```python
from build123d import *

# Parameters (mm, degrees)
BOSS_EXTRUDE1_DEPTH                = 25.4
FILLET1_R                          = 25.4
F_1_4_0_25_DIAMETER_SLOT1_DEPTH    = 25.4
F_1_16_0_0625_DIAMETER_HOLE1_D     = 1.5875
F_1_16_0_0625_DIAMETER_HOLE1_DEPTH = 12.7
F_1_16_0_0625_DIAMETER_HOLE1_TIP   = 0.476933116


# Read off the part's stored shape, not the designer's step: 1/4 (0.25) Diameter Slot1
with BuildPart() as part:
    # Sketch1 → Boss-Extrude1 (new body)
    with BuildSketch(Plane.XY):
        Polygon((-203.2, 0), (203.2, 0), (173.589463707, -63.5), (-173.589463707, -63.5), align=None)
    extrude(amount=BOSS_EXTRUDE1_DEPTH)

    # Fillet1
    fillet1_edges = [part.edges().sort_by_distance(p)[0] for p in [
        (173.589463707, -63.5, 12.7),
        (-173.589463707, -63.5, 12.7),
    ]]
    fillet(fillet1_edges, radius=FILLET1_R)

    # 1/4 (0.25) Diameter Slot1 outline → 1/4 (0.25) Diameter Slot1 (cut)
    with BuildSketch(Plane.XY):
        with BuildLine():
            Line((-149.225, -41.275), (149.225, -41.275))
            ThreePointArc((149.225, -41.275), (152.4, -38.1), (149.225, -34.925))
            Line((149.225, -34.925), (-149.225, -34.925))
            ThreePointArc((-149.225, -34.925), (-152.4, -38.1), (-149.225, -41.275))
        make_face()
    extrude(amount=F_1_4_0_25_DIAMETER_SLOT1_DEPTH, mode=Mode.SUBTRACT)

    # 1/16 (0.0625) Diameter Hole1
    with Locations(Plane(origin=(0, 0, 0), x_dir=(1, 0, 0), z_dir=(0, 1, 0))):
        with Locations((-152.4, -12.7), (-101.6, -12.7), (-50.8, -12.7), (0, -12.7), (50.8, -12.7), (101.6, -12.7), (152.4, -12.7)):
            Hole(F_1_16_0_0625_DIAMETER_HOLE1_D / 2, depth=F_1_16_0_0625_DIAMETER_HOLE1_DEPTH)
            with Locations((0, 0, -(F_1_16_0_0625_DIAMETER_HOLE1_DEPTH + F_1_16_0_0625_DIAMETER_HOLE1_TIP / 2))):  # 118° drill point
                Cone(0, F_1_16_0_0625_DIAMETER_HOLE1_D / 2, F_1_16_0_0625_DIAMETER_HOLE1_TIP, mode=Mode.SUBTRACT)


solid = part.part
```
Input: part model. Units: mm. Frame: model coordinates. A direction names the side the tool comes from. Give positions to 0.01 mm unless a question says otherwise; leave off trailing zeros. Order: outer loops, then holes, each group sorted by start corner. A loop starts at its lowest first (then second) coordinate and runs counter-clockwise, first axis right, second up. Notation, with made-up numbers: M 1.5,-17.75 L 60.5,-17.75 A12 cw 60.5,-1.75 Z; hole C 87.5,14 d2. An arc over 180 degrees is marked long. One line per question, with ' | ' between items.
1) Access query for faces 4 (the face through (152.4, -38.2, 12.5)), 5 (the face through (3, -31, 0)). Directions: +Z, -Z, +X, -X, +Y, -Y. A direction counts if a zero-diameter tool reaches every point of the face in a straight line with its end or side. Return the directions, or none.
Filled in:
face 4: +Z, -Z | face 5: -Z, +X, -X, +Y, -Y
2) Draft query along Y for faces 1 (the face through (-3, 0, 13)), 2 (the face through (191.97, -24.08, 12.52)), 3 (the face through (-2, -41.275, 13)). Return one class per face: pulls with the +Y half, pulls with the -Y half, needs draft (parallel to the pull), parting line crosses it, or undercut.
Filled in:
face 1: pulls with the +Y half | face 2: pulls with the -Y half | face 3: undercut
3) Contact query for flat-ended pins moving along their axis: P1, Ø5, axis at y = -50, z = 10, coming from the +X side; P2, Ø1, axis at y = -21.5, z = 18, coming from the -X side; P3, Ø1, axis at x = 50.8, z = 12.7, coming from the +Y side. Output: stop coordinate, or through.
Filled in:
P1: stops at x = 181.05 | P2: stops at x = -193.41 | P3: stops at y = -12.88
4) Section D-D on x = -167.5. Output: boundary loops of the cut face in (y, z).
Filled in:
outline: M -61.41,0 L 0,0 L 0,25.4 L -61.41,25.4 Z
5) Section A-A on x = -20. Output: boundary loops of the cut face in (y, z) (3 decimals), and give its area (3 significant figures).
Filled in:
outline: M -63.5,0 L -41.275,0 L -41.275,25.4 L -63.5,25.4 Z; M -34.925,0 L 0,0 L 0,25.4 L -34.925,25.4 Z | area: 1,450 mm2
6) Ray query, L1, parallel to Y at x = -111, z = 22.5 (3 decimals); L2, parallel to Z at x = 152.4, y = -5; L3, parallel to Z at x = -101, y = -6. Return the intervals inside material, ascending.
Filled in:
L1: y = -63.5 to -41.275, -34.925 to 0 | L2: z = 0 to 11.91, 13.49 to 25.4 | L3: z = 0 to 12.18, 13.22 to 25.4
7) Section C-C on y = -22.5. Output: boundary loops of the cut face in (x, z), and give its area (3 significant figures).
Filled in:
outline: M -192.71,0 L 192.71,0 L 192.71,25.4 L -192.71,25.4 Z | area: 9,790 mm2
